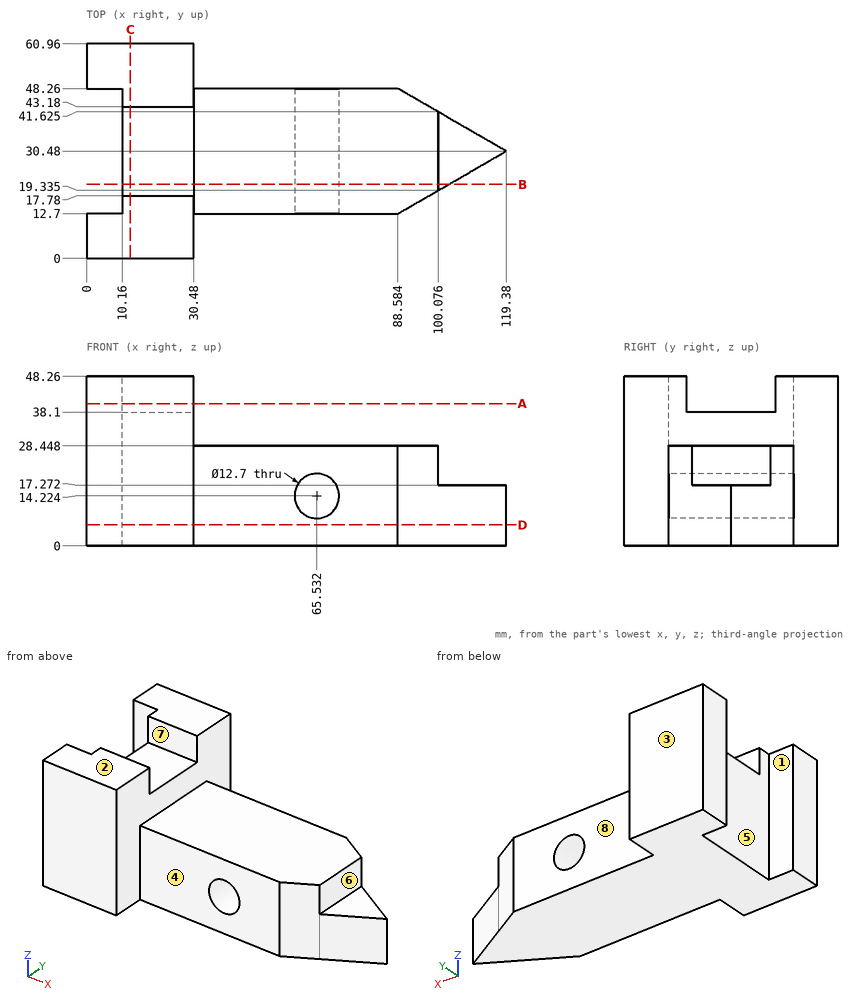
Geometry: see drawing. Coordinates: mm, zero at the bounding-box minimum. A direction names the side the tool comes from. Coordinates: 2 decimals unless noted, no trailing zeros. Write each loop counter-clockwise with the first axis right and the second up, starting at its lowest first coordinate (ties: lowest second). Pieces come first, ordered by that corner, then holes. Notation, with made-up numbers: (-17.5, 36.25) - (18.5, 36.25) arc R26 ccw to (18.5, 53.25) - close; hole circle Ø10 at (-29.75, -24). An arc over 180 degrees is marked (long way). Put each result on its own line as item: value. Start each with the question number.
1) Cut plane D-D (z = 6). Return the cut outline in (x, y) (1 decimal).
2) Ray query, L1, parallel to Z at x = 66, y = 34; L2, parallel to Z at x = 33, y = 35.5; L3, parallel to X at y = 44, z = 37.5. Return the intervals inside material, ascending.
3) Reachability of the marked faces 4, 5, 6, 7 and 8 from +Z, -Z, +X, -X, +Y, -Y: full face, straight path, thin tool, end or side. Return the list, or none.
4) Contact query for flat-ended pins moving along their axis: pin 1 (4 mm diameter, centred on x = 34.5, z = 5.5, fed in from +Y); pin 2 (14 mm diameter, centred on x = 55, z = 13, fed in from -Y); pin 3 (6 mm diameter, centred on x = 37, y = 36.5, fed in from +Z). Output: stop coordinate, or through.
5) Cut plane C-C (x = 12.5). Return the cut outline in (y, z), plus the area to 3 significant figures.
6) Cut plane B-B (y = 21). Return the cut outline in (x, z), plus the area to 3 significant figures.
7) Mould query, pull axis Y, two halves, no side actions, for the marked faces 1, 2 and 3. Classes: pulls with the +Y half, pulls with the -Y half, needs draft (parallel to the pull), parting line crosses it, or undercut.
8) Cut plane A-A (z = 40.5). Return the cut outline in (x, y), plus the area to 3 significant figures.
Resolved:
1. outline: (0, 0) - (30.5, 0) - (30.5, 12.7) - (88.6, 12.7) - (119.4, 30.5) - (88.6, 48.3) - (30.5, 48.3) - (30.5, 61) - (0, 61) - (0, 48.3) - (10.2, 48.3) - (10.2, 12.7) - (0, 12.7) - close
2. L1: z = 0 to 7.89, 20.56 to 28.45
2. L2: z = 0 to 28.45
2. L3: x = 10.16 to 30.48
3. face 4: +Z, -Z, +X, -Y
3. face 5: +Z, -Z, -X
3. face 6: +Z, +X, +Y, -Y
3. face 7: +Z, +X, -X
3. face 8: +Z, -Z, +X, +Y
4. pin 1: stops at y = 48.26
4. pin 2: stops at y = 12.7
4. pin 3: stops at z = 28.45
5. outline: (0, 0) - (60.96, 0) - (60.96, 48.26) - (43.18, 48.26) - (43.18, 38.1) - (17.78, 38.1) - (17.78, 48.26) - (0, 48.26) - close
5. area: 2,680 mm2
6. outline: (10.16, 0) - (102.96, 0) - (102.96, 17.27) - (100.08, 17.27) - (100.08, 28.45) - (30.48, 28.45) - (30.48, 38.1) - (10.16, 38.1) - close; hole circle Ø12.7 at (65.53, 14.22)
6. area: 2,680 mm2
7. face 1: undercut
7. face 2: needs draft
7. face 3: pulls with the +Y half
8. outline: (0, 0) - (30.48, 0) - (30.48, 17.78) - (10.16, 17.78) - (10.16, 12.7) - (0, 12.7) - close; (0, 48.26) - (10.16, 48.26) - (10.16, 43.18) - (30.48, 43.18) - (30.48, 60.96) - (0, 60.96) - close
8. area: 981 mm2
